Source: CAD feature listing. Evaluate the final solid. Frame: model axes, mm. A direction names the side the tool comes from. Give positions to 0.01 mm unless a question says otherwise; leave off trailing zeros. Order: outer loops, then holes, each group sorted by start corner. A loop starts at its lowest first (then second) coordinate and runs counter-clockwise, first axis right, second up. Notation, with made-up numbers: (5, 17.25) -> (26, 17.25) arc R12 ccw to (26, 36.25) -> close; hole circle Ø6 at (0, 67.25). An arc over 180 degrees is marked (long way). Answer in a Markdown table with one row per item.
```python
from build123d import *

# Parameters (mm, degrees)
F0_W        = 210
F0_H        = 80
F1_DEPTH    = 3
F2_R        = 2
F3_DEPTH    = 25
F4_W        = 10
F4_H        = 10
F4_R        = 2
F5_DEPTH    = 2
F6_W        = 5
F6_H        = 60
F7_DEPTH    = 25
F8_T1_DEPTH = 3
F8_T3_DEPTH = 7
F8_T5_DEPTH = 8
F8_T7_DEPTH = 15


# Not quite as in the source:
# - a fillet or chamfer that OpenCascade refuses, or shapes differently, is made with other operations: its cross-section is extruded or revolved along the edge and cut away or added


with BuildPart() as f1:
    # F0 (on Front) → F1 (new body)
    with BuildSketch(Plane.XZ):
        Rectangle(F0_W, F0_H)
    extrude(amount=F1_DEPTH)

    # F2 (on face) → F3 (cut)
    with BuildSketch(Plane.XZ.offset(3)):
        with Locations((-100.000000149, 35.000000149)):
            Circle(F2_R)
        with Locations((-100.000000149, -35.000000149)):
            Circle(F2_R)
        with Locations((100.000000149, -35.000000149)):
            Circle(F2_R)
        with Locations((100.000000149, 35.000000149)):
            Circle(F2_R)
    extrude(amount=-F3_DEPTH, mode=Mode.SUBTRACT)

    # F4 (on face) → F5 (join)
    with BuildSketch(Plane.XZ.offset(3)):
        with Locations((-100, 35)):
            Rectangle(F4_W, F4_H)
        with Locations((-100.000000149, 35.000000149)):
            Circle(F4_R, mode=Mode.SUBTRACT)
        with Locations((-100, -35)):
            Rectangle(F4_W, F4_H)
        with Locations((-100.000000149, -35.000000149)):
            Circle(F4_R, mode=Mode.SUBTRACT)
        with Locations((100, -35)):
            Rectangle(F4_W, F4_H)
        with Locations((100.000000149, -35.000000149)):
            Circle(F4_R, mode=Mode.SUBTRACT)
        with Locations((100, 35)):
            Rectangle(F4_W, F4_H)
        with Locations((100.000000149, 35.000000149)):
            Circle(F4_R, mode=Mode.SUBTRACT)
    extrude(amount=F5_DEPTH)

    # F6 (on face) → F7 (cut)
    with BuildSketch(Plane.XZ.offset(3)):
        Polygon((95, 35), (-95, 35), (-95, 30), (-95, -30), (-95, -35), (95, -35), (95, -30), (95, 30), align=None)
        with Locations((-97.5, 0)):
            Rectangle(F6_W, F6_H)
        with Locations((97.5, 0)):
            Rectangle(F6_W, F6_H)
    extrude(amount=-F7_DEPTH, mode=Mode.SUBTRACT)

    # F8: fillet of radius 2 on 15 edges, made by hand

    # F8_s2 → F8_t1 (join)
    with BuildSketch(Plane.XZ):
        with BuildLine():
            ThreePointArc((-100, 28), (-99.4142135624, 29.4142135624), (-98, 30))
            Line((-98, 30), (-100, 30))
            Line((-100, 30), (-100, 28))
        make_face()
        with BuildLine():
            ThreePointArc((-95, 33), (-94.4142135624, 34.4142135624), (-93, 35))
            Line((-93, 35), (-95, 35))
            Line((-95, 35), (-95, 33))
        make_face()
        with BuildLine():
            ThreePointArc((-98, -30), (-99.4142135624, -29.4142135624), (-100, -28))
            Line((-100, -28), (-100, -30))
            Line((-100, -30), (-98, -30))
        make_face()
        with BuildLine():
            ThreePointArc((-93, -35), (-94.4142135624, -34.4142135624), (-95, -33))
            Line((-95, -33), (-95, -35))
            Line((-95, -35), (-93, -35))
        make_face()
        with BuildLine():
            ThreePointArc((95, 33), (94.4142135624, 34.4142135624), (93, 35))
            Line((93, 35), (95, 35))
            Line((95, 35), (95, 33))
        make_face()
        with BuildLine():
            ThreePointArc((100, 28), (99.4142135624, 29.4142135624), (98, 30))
            Line((98, 30), (100, 30))
            Line((100, 30), (100, 28))
        make_face()
        with BuildLine():
            ThreePointArc((95, -33), (94.4142135624, -34.4142135624), (93, -35))
            Line((93, -35), (95, -35))
            Line((95, -35), (95, -33))
        make_face()
        with BuildLine():
            ThreePointArc((100, -28), (99.4142135624, -29.4142135624), (98, -30))
            Line((98, -30), (100, -30))
            Line((100, -30), (100, -28))
        make_face()
    extrude(amount=F8_T1_DEPTH)

    # F8_s4 → F8_t3 (cut)
    with BuildSketch(Plane.XZ.offset(3)):
        with BuildLine():
            ThreePointArc((-95, 32), (-95.5857864376, 30.5857864376), (-97, 30))
            Line((-97, 30), (-95, 30))
            Line((-95, 30), (-95, 32))
        make_face()
        with BuildLine():
            ThreePointArc((-97, -30), (-95.5857864376, -30.5857864376), (-95, -32))
            Line((-95, -32), (-95, -30))
            Line((-95, -30), (-97, -30))
        make_face()
        with BuildLine():
            ThreePointArc((95, 32), (95.5857864376, 30.5857864376), (97, 30))
            Line((97, 30), (95, 30))
            Line((95, 30), (95, 32))
        make_face()
    extrude(amount=F8_T3_DEPTH, mode=Mode.SUBTRACT)

    # F8_s6 → F8_t5 (cut)
    with BuildSketch(Plane.XZ.offset(-5)):
        with BuildLine():
            ThreePointArc((-95, 32), (-95.5857864376, 30.5857864376), (-97, 30))
            Line((-97, 30), (-95, 30))
            Line((-95, 30), (-95, 32))
        make_face()
        with BuildLine():
            ThreePointArc((-97, -30), (-95.5857864376, -30.5857864376), (-95, -32))
            Line((-95, -32), (-95, -30))
            Line((-95, -30), (-97, -30))
        make_face()
        with BuildLine():
            ThreePointArc((95, 32), (95.5857864376, 30.5857864376), (97, 30))
            Line((97, 30), (95, 30))
            Line((95, 30), (95, 32))
        make_face()
    extrude(amount=F8_T5_DEPTH, mode=Mode.SUBTRACT)

    # F8_s8 → F8_t7 (cut)
    with BuildSketch(Plane.XZ.offset(-5)):
        with BuildLine():
            ThreePointArc((95, -32), (95.5857864376, -30.5857864376), (97, -30))
            Line((97, -30), (95, -30))
            Line((95, -30), (95, -32))
        make_face()
    extrude(amount=F8_T7_DEPTH, mode=Mode.SUBTRACT)


solid = f1.part
```
(1) Section query C-C (y = -0.8). Give the number of separate pieces and of enclosed holes in the cut face, plus the area to 3 significant figures.
A:
| item | result |
|---|---|
| separate pieces | 1 |
| enclosed holes | 5 |
| area | 2,850 mm^2 |
(2) Ray query, probe 1 along Z at (x, y) = (100, -4.45); probe 2 along Z at (x, y) = (-40.5, -2.15); probe 3 along X at (y, z) = (-0.75, -17.5). Return the intervals inside material, ascending.
A:
| item | result |
|---|---|
| probe 1 | z = -40 to -37, -33 to -30, 30 to 33, 37 to 40 |
| probe 2 | z = -40 to -35, 35 to 40 |
| probe 3 | x = -105 to -100, 100 to 105 |
(3) Pull-direction query (Z, two-part tool) for faces 4 (the flat face through (-101, -4, -30)), 5 (the flat face through (-1, -1, 40)), 6 (the flat face through (-8.3, 0, -35.4)); classes: +Z half, -Z half, draft (parallel to the pull), parting line (faces both ways), or undercut.
A:
| item | result |
|---|---|
| face 4 | undercut |
| face 5 | +Z half |
| face 6 | draft |
(4) Section query A-A (x = -39). Return the cut outline in (y, z), plus the area to 3 significant figures.
A:
| item | result |
|---|---|
| outline | (-3, -40) -> (0, -40) -> (0, -35) -> (-3, -35) -> close; (-3, 35) -> (0, 35) -> (0, 40) -> (-3, 40) -> close |
| area | 30.0 mm^2 |
(5) Access query for faces 1 (the flat face through (-95, -4, -36)), 2 (the flat face through (-103, -3, 0)), 3 (the flat face through (99.9, -5, -37.2)). Directions: +Z, -Z, +X, -X, +Y, -Y. A direction counts if a zero-diameter tool reaches every point of the face in a straight line with its end or side. Return the directions, or none.
A:
| item | result |
|---|---|
| face 1 | -Y |
| face 2 | +X, -X, -Y |
| face 3 | +Z, -Z, +X, -X, -Y |
(6) First-contact query: pin 1 Ø2.5 at (x, z) = (-42, 37) entering from -Y; pin 2 Ø2.5 at (x, z) = (-100, 35) entering from +Y. Flat tips, straight axial feed; report the tip coordinate or a pass-through.
A:
| item | result |
|---|---|
| pin 1 | stops at y = -3 |
| pin 2 | passes through |
(7) Section query B-B (z = 18.5). Return the cut outline in (x, y).
A:
| item | result |
|---|---|
| outline | (-105, -3) -> (-100, -3) -> (-100, 0) -> (-105, 0) -> close; (100, -3) -> (105, -3) -> (105, 0) -> (100, 0) -> close |
